from build123d import *

# Parameters (mm, degrees)
ESBO_O1_W                = 130.25
ESBO_O1_H                = 75
RESSALTO_EXTRUS_O1_DEPTH = 2
ESBO_O2_W                = 75
ESBO_O2_H                = 18
RESSALTO_EXTRUS_O2_DEPTH = 2
ESBO_O3_R                = 2.5
CORTE_EXTRUS_O1_DEPTH    = 135.25


with BuildPart() as part:
    # Esboço1 → Ressalto-extrusão1 (new body)
    with BuildSketch(Plane(origin=(0, 0, 0), x_dir=(1, 0, 0), z_dir=(0, 1, 0))):
        Rectangle(ESBO_O1_W, ESBO_O1_H)
    extrude(amount=RESSALTO_EXTRUS_O1_DEPTH)

    # Esboço2 → Ressalto-extrusão2 (add)
    with BuildSketch(Plane(origin=(65.125, 0, 0), x_dir=(0, 0, -1), z_dir=(1, 0, 0))):
        with Locations((0, 9)):
            Rectangle(ESBO_O2_W, ESBO_O2_H)
    ressalto_extrus_o2 = extrude(amount=RESSALTO_EXTRUS_O2_DEPTH)

    # Espelhar1: Ressalto-extrusão2 across plane
    add(ressalto_extrus_o2.mirror(Plane(origin=(0, 0, 0), x_dir=(0, 0, 1), z_dir=(1, 0, 0))))

    # Esboço3 → Corte-extrusão1 (cut, through all)
    with BuildSketch(Plane.ZY.offset(67.125)):
        with Locations((-28.5, 10)):
            Circle(ESBO_O3_R)
        with Locations((28.5, 10)):
            Circle(ESBO_O3_R)
    extrude(amount=-CORTE_EXTRUS_O1_DEPTH, mode=Mode.SUBTRACT)


solid = part.part
Here's how the part is built. I have some questions about the finished solid (model axes, mm). A direction names the side the tool comes from. Coordinates: 2 decimals unless noted, no trailing zeros. Loops run counter-clockwise (first coordinate to the right, second up) from the corner with the lowest first, then second, coordinate; pieces in that order, holes last.
1. For faces 1 (the flat face through (67.125, 9, 1)), 2 (the flat face through (-65.125, 10, 1)), which set-ups out of +Z, -Z, +X, -X, +Y, -Y let a thin tool reach every point of the face, with its end or its side?
2. Imagine slicing it at C-C, the plane y = 4. Please give me the cut outline in (x, z) (3 decimals), and give its area (3 significant figures).
3. Imagine slicing it at B-B, the plane z = -28.5. Please give me the cut outline in (x, y) (3 decimals), and give its area (4 significant figures).
4. Imagine slicing it at D-D, the plane z = 16. Please give me the cut outline in (x, y) (3 decimals), and give its area (4 significant figures).
5. For P1, Ø3, axis at x = 42.5, z = 22.5, coming from the +Y side, with a flat end and sliding along its axis, tell me the tip position at first contact or that it passes through.
6. If we mould it in two halves opening along Y, with no side actions, what happens to faces 3 (the cylindrical face through (66.11, 7.56, -29.04)), 4 (the flat face through (65.125, 10, 1)), 5 (the flat face through (1, 0, 1))? For each: pulls with the +Y half, pulls with the -Y half, needs draft (parallel to the pull), parting line crosses it, or undercut.
7. I need wall thicknesses on L1, parallel to X at y = 7.5, z = 9 (3 decimals); L2, parallel to Y at x = 36, z = -7.5; L3, parallel to Y at x = 65.8, z = -28.5. Which ranges of each line are inside material? Lowest first, please.
8. Imagine slicing it at A-A, the plane y = 10. Please give me the cut outline in (x, z) (3 decimals).
Taken from the geometry:
1. face 1: +Z, -Z, +X, +Y, -Y
1. face 2: +Z, -Z, +Y
2. outline: (-67.125, -37.5) - (-65.125, -37.5) - (-65.125, 37.5) - (-67.125, 37.5) - close; (65.125, -37.5) - (67.125, -37.5) - (67.125, 37.5) - (65.125, 37.5) - close
2. area: 300 mm2
3. outline: (-67.125, 0) - (67.125, 0) - (67.125, 7.5) - (65.125, 7.5) - (65.125, 2) - (-65.125, 2) - (-65.125, 7.5) - (-67.125, 7.5) - close; (-67.125, 12.5) - (-65.125, 12.5) - (-65.125, 18) - (-67.125, 18) - close; (65.125, 12.5) - (67.125, 12.5) - (67.125, 18) - (65.125, 18) - close
3. area: 312.5 mm2
4. outline: (-67.125, 0) - (67.125, 0) - (67.125, 18) - (65.125, 18) - (65.125, 2) - (-65.125, 2) - (-65.125, 18) - (-67.125, 18) - close
4. area: 332.5 mm2
5. P1: stops at y = 2
6. face 3: undercut
6. face 4: needs draft
6. face 5: pulls with the -Y half
7. L1: x = -67.125 to -65.125, 65.125 to 67.125
7. L2: y = 0 to 2
7. L3: y = 0 to 7.5, 12.5 to 18
8. outline: (-67.125, -37.5) - (-65.125, -37.5) - (-65.125, -31) - (-67.125, -31) - close; (-67.125, -26) - (-65.125, -26) - (-65.125, 26) - (-67.125, 26) - close; (-67.125, 31) - (-65.125, 31) - (-65.125, 37.5) - (-67.125, 37.5) - close; (65.125, -37.5) - (67.125, -37.5) - (67.125, -31) - (65.125, -31) - close; (65.125, -26) - (67.125, -26) - (67.125, 26) - (65.125, 26) - close; (65.125, 31) - (67.125, 31) - (67.125, 37.5) - (65.125, 37.5) - close
